Autodesk Inventor part; units mm, degrees
ref_plane "YZ Plane" through (0, 0, 0) normal (1, 0, 0) x (0, 1, 0)
ref_plane "XZ Plane" through (0, 0, 0) normal (0, 1, 0) x (-1, 0, 0)
ref_plane "XY Plane" through (0, 0, 0) normal (0, 0, 1) x (1, 0, 0)
sketch "Эскиз1" plane through (0, 0, 0) normal (0, 0, 1) x (1, 0, 0)
  circle A0 centre (0, 0) radius 2.1
  line L0 (-5, 14.35) -> (5, 14.35)
  line L1 (5, 14.35) -> (5, -14.35)
  line L2 (5, -14.35) -> (-5, -14.35)
  line L3 (-5, -14.35) -> (-5, 14.35)
  line L4 (-5, 14.35) -> (5, -14.35) construction
  line L5 (5, 14.35) -> (-5, -14.35) construction
  line L6 (-5, 7) -> (5, 7)
  dimension "d0" = 4.2
  dimension "d2" = 10
  dimension "d3" = 28.7
  dimension "d4" = 7
extrude "Выдавливание1" add sketch "Эскиз1" along normal blind 3.2 contours L6 L1 L2 L3
sketch "Эскиз2" plane through (0, 0, 3.2) normal (0, 0, 1) x (1, 0, 0)
  line L0 (5, -14.35) -> (5, 7)
  line L1 (5, -14.35) -> (-5, -14.35)
  line L2 (-5, -14.35) -> (-5, -11.15)
  line L3 (-5, -11.15) -> (5, -11.15)
  line L4 (5, -11.15) -> (5, -14.35)
  point P0 (0, 0)
  point P1 (5, -11.15)
  dimension "d7" = 10
  dimension "d8" = 3.2
extrude "Выдавливание2" add sketch "Эскиз2" along normal blind 13
fillet "Сопряжение1" radius 3 1 edges at (0, -11.15, 3.2)
sketch "Эскиз3" plane through (-5, -11.15, 16.2) normal (0, 1, 0) x (1, 0, 0)
  line L0 (0, 10) -> (10, 10)
  line L1 (5, 10) -> (5, 0)
  line L2 (0, 0) -> (10, 0)
  circle A0 centre (5, 5) radius 2.1
  point P0 (5, 16.2)
  dimension "d12" = 4.2
extrude "Выдавливание3" cut sketch "Эскиз3" against normal blind 13
sketch "Эскиз4" plane through (0, 0, 3.2) normal (0, 0, 1) x (1, 0, 0)
  circle A0 centre (37.4046, 25.4735) radius 2.6917
  line L0 (35.1798, 23.9584) -> (0, 0)
  line L1 (29.7757, 32.3768) -> (-5, 8.6936)
  line L2 (-5, 7) -> (-5, -8.15)
  line L3 (-5, 7) -> (-5, 8.6936)
  line L4 (-5, -14.35) -> (5, -14.35)
  line L5 (5, -14.35) -> (5, -11.15)
  line L6 (5, -11.15) -> (-5, -11.15)
  line L7 (-5, -11.15) -> (-5, -14.35)
  line L8 (37.4046, 25.4735) -> (37.4046, -14.35)
  line L9 (45.4046, 24.1114) -> (45.4046, -14.35)
  arc A1 (45.4046, 24.1114) -> (29.7757, 32.3768) centre (35.4046, 24.1114) ccw
  line L10 (-5, -14.35) -> (45.4046, -14.35)
  circle A2 centre (37.4046, 25.4735) radius 2.25
  line L11 (-5, 8.6936) -> (-5, -14.35)
  circle A3 centre (0, 0) radius 2.1
  dimension "d15" = 10
  dimension "d16" = 8
  dimension "d17" = 10
  dimension "d18" = 4.5
extrude "Выдавливание4" add sketch "Эскиз4" against normal up to surface (3.2 mm away) contours A0 | A1 L9 L10 L5 L6 L11 L2 L3 L1
fillet "Сопряжение2" radius 3 1 edges at (5, -11.25, 3.2)
ref_plane "РабПлоскость1" through (20.202, -14.35, 16.2) normal (-1, 0, 0) x (0, 0, 1)
mirror "Зеркальное отражение1" about plane through (20.202, -14.35, 16.2) normal (-1, 0, 0) of "Выдавливание2", "Выдавливание3", "Сопряжение1", "Сопряжение2"
properties part number "мертвое колесо 3"
For this review, take the finished solid that the model builds, in its own axes (mm). A direction names the side the tool comes from. Give positions to 0.01 mm unless a question says otherwise; leave off trailing zeros. Order: outer loops, then holes, each group sorted by start corner. A loop starts at its lowest first (then second) coordinate and runs counter-clockwise, first axis right, second up.
1) Take a section at A-A (y = 0). Give the boundary of the cut face in (x, z), then the cut area to 3 significant figures.
2) Take a section at D-D (z = 4.5). Give the boundary of the cut face in (x, y).
3) Wall thickness on line 1 (Z direction, x = 0, y = -12.8); line 2 (Z direction, x = 16, y = 15); line 3 (Z direction, x = 38.5, y = -12): over which ranges is each line inside the solid? List them lowest first.
4) For faces 1 (the face through (34.15, -11.9, 3.76)), 2 (the face through (-5, -7, 3)), 3 (the face through (43, -11.15, 11)), list the 3-axis set-ups (+Z, -Z, +X, -X, +Y, -Y) from which the entire face can be reached by the end or side of a thin tool; tool diameter is ignored.
5) The part is to be moulded in two halves that separate along Y. For faces 4 (the face through (35.157, 25.572, 1.622)), 5 (the face through (40.26, -10.25, 4.06)), 6 (the face through (5, -13, 11)), say which applies: released by +Y, released by -Y, zero draft, split by the parting line, or undercut.
6) Take a section at B-B (z = 12.5). Give the boundary of the cut face in (x, y), then the cut area to 3 significant figures.
7) Insertion check: pin 1 (6 mm diameter, centred on x = 21.5, y = -8.5, fed in from +Z). The pin has a flat end and moves straight along its axis. Give the tip position at first contact, or say it passes through.
8) Take a section at C-C (x = 0). Give the boundary of the cut face in (y, z).
Derived:
1. outline: (-5, 0) - (-2.1, 0) - (-2.1, 3.2) - (-5, 3.2) - close; (2.1, 0) - (45.4, 0) - (45.4, 3.2) - (2.1, 3.2) - close
1. area: 148 mm2
2. outline: (-5, -14.35) - (5.53, -14.35) - (5.53, -10.62) - (-5, -10.62) - close; (34.88, -14.35) - (45.4, -14.35) - (45.4, -10.62) - (34.88, -10.62) - close
3. line 1: z = 0 to 9.1, 13.3 to 16.2
3. line 2: z = 0 to 3.2
3. line 3: z = 0 to 10.31, 12.09 to 16.2
4. face 1: +Z, +Y, -Y
4. face 2: +Z, -Z, -X, +Y, -Y
4. face 3: +Z, +X, -X, +Y
5. face 4: undercut
5. face 5: released by +Y
5. face 6: zero draft
6. outline: (-5, -14.35) - (-1.65, -14.35) - (-1.65, -11.15) - (-5, -11.15) - close; (1.65, -14.35) - (5, -14.35) - (5, -11.15) - (1.65, -11.15) - close; (35.4, -14.35) - (38.75, -14.35) - (38.75, -11.15) - (35.4, -11.15) - close; (42.05, -14.35) - (45.4, -14.35) - (45.4, -11.15) - (42.05, -11.15) - close
6. area: 42.9 mm2
7. pin 1: stops at z = 3.2
8. outline: (-14.35, 0) - (-2.1, 0) - (-2.1, 3.2) - (-8.15, 3.2) arc R3 cw to (-11.15, 6.2) - (-11.15, 9.1) - (-14.35, 9.1) - close; (-14.35, 13.3) - (-11.15, 13.3) - (-11.15, 16.2) - (-14.35, 16.2) - close; (2.1, 0) - (12.1, 0) - (12.1, 3.2) - (2.1, 3.2) - close
